Check sheet for the modelled part. Datum: model origin and axes. Units: mm. A direction names the side the tool comes from. Give positions to 0.01 mm unless a question says otherwise; leave off trailing zeros. Write each loop counter-clockwise with the first axis right and the second up, starting at its lowest first coordinate (ties: lowest second). Pieces come first, ordered by that corner, then holes. Notation, with made-up numbers: M 64,85.5 L 111,85.5 A35 cw 111,117.5 Z; hole C 85.25,14 d8. An arc over 180 degrees is marked long. Use CSV: the item, a comma, the result in double quotes. Start each with the question number.
1. Cross-section at A-A, the plane y = 0. Enter the section's corners in (x, z).
2. Cross-section at C-C, the plane z = 34.3. State how many separate pieces and enclosed holes the cut face has, and give its area (3 significant figures).
3. Mould release check, pull along X, two halves, no side actions. Record for faces 3 (the face through (47.7, -40.23, 34.39)), 4 (the face through (44, 0.07, 34.61)), 5 (the face through (-47.7, 40.23, 34.39)), 6 (the face through (44.39, -36.99, 34.61)): +X half, -X half, draft (parallel to the pull), parting line (faces both ways), or undercut.
4. Depth check by flat-ended pin: P1, Ø1.8, axis at x = -45.5, y = 38, coming from the -Z side; P2, Ø0.9, axis at y = 34, z = 35.5, coming from the +X side. Enter the tip coordinate at first touch or a pass-through.
5. Access from +Z, -Z, +X, -X, +Y, -Y to the whole of each face (thin tool, end or side, straight path). Record for faces 1 (the face through (-4, -36, 34.8)), 2 (the face through (-47, 0.07, 34.61)).
6. Scan lines: line 1 (Y direction, x = 45.5, z = 35.35); line 2 (Y direction, x = -45.5, z = 34.85); line 3 (Y direction, x = -37.5, z = 35.45). Record each from-to range of solid material in increasing order.
7. Cross-section at B-B, the plane y = 29. Enter the section's corners in (x, z).
8. Cross-section at D-D, the plane x = -10. Enter the section's corners in (y, z), and give its area (3 significant figures).
from build123d import *

# Parameters (mm, degrees)
PAD011_DEPTH         = 0.8
SKETCH019_W          = 92
SKETCH019_H          = 77
SKETCH019_W_2        = 90
SKETCH019_H_2        = 75
PAD012_DEPTH         = 1.6
SKETCH018_R          = 1.5
POCKET007_DEPTH      = 1.6
POCKET007_DEPTH_BACK = 0.8


with BuildPart() as part:
    # Sketch017 (on XY_Plane002 of Origin004) → Pad011 (new body)
    with BuildSketch(Plane.XY):
        with BuildLine():
            Line((48.3, -38.8), (48.3, 38.8))
            ThreePointArc((48.3, 38.8), (47.714214, 40.214214), (46.3, 40.8))
            Line((46.3, 40.8), (-46.3, 40.8))
            ThreePointArc((-46.3, 40.8), (-47.714214, 40.214214), (-48.3, 38.8))
            Line((-48.3, 38.8), (-48.3, -38.8))
            ThreePointArc((-48.3, -38.8), (-47.714214, -40.214214), (-46.3, -40.8))
            Line((-46.3, -40.8), (46.3, -40.8))
            ThreePointArc((46.3, -40.8), (47.714214, -40.214214), (48.3, -38.8))
        make_face()
        Polygon((-42.5, 35), (42.5, 35), (42.5, -17), (37.5, -17), (37.5, -35), (-37.5, -35), (-37.5, -17), (-42.5, -17), align=None, mode=Mode.SUBTRACT)
    extrude(amount=PAD011_DEPTH)

    # Sketch019 (on XY_Plane002 of Origin004) → Pad012 (join)
    with BuildSketch(Plane.XY):
        Rectangle(SKETCH019_W, SKETCH019_H)
        Rectangle(SKETCH019_W_2, SKETCH019_H_2, mode=Mode.SUBTRACT)
    extrude(amount=PAD012_DEPTH)

    # Sketch018 (on XY_Plane002 of Origin004) → Pocket007 (cut, two sides)
    with BuildSketch(Plane.XY) as pocket007_sk:
        with Locations((-45.5, 38)):
            Circle(SKETCH018_R)
        with Locations((-15.166667, 38)):
            Circle(SKETCH018_R)
        with Locations((15.166667, 38)):
            Circle(SKETCH018_R)
        with Locations((45.5, 29)):
            Circle(SKETCH018_R)
        with Locations((45.5, 0)):
            Circle(SKETCH018_R)
        with Locations((45.5, -38)):
            Circle(SKETCH018_R)
        with Locations((15.166667, -38)):
            Circle(SKETCH018_R)
        with Locations((-15.166667, -38)):
            Circle(SKETCH018_R)
        with Locations((-45.5, -38)):
            Circle(SKETCH018_R)
        with Locations((-45.5, 0)):
            Circle(SKETCH018_R)
    extrude(amount=POCKET007_DEPTH, mode=Mode.SUBTRACT)
    extrude(pocket007_sk.sketch, amount=-POCKET007_DEPTH_BACK, mode=Mode.SUBTRACT)


with BuildPart() as part_1:
    # Body002 placement: moved
    add(part.part.moved(Location((0, 0, 34))))


solid = part_1.part
Worked answers:
1,outline,"M -48.3,34 L -47,34 L -47,34.8 L -48.3,34.8 Z; M -44,34 L -42.5,34 L -42.5,34.8 L -44,34.8 Z; M 42.5,34 L 44,34 L 44,34.8 L 42.5,34.8 Z; M 47,34 L 48.3,34 L 48.3,34.8 L 47,34.8 Z"
2,separate pieces,"1"
2,enclosed holes,"11"
2,area,"2,040 mm^2"
3,face 3,"+X half"
3,face 4,"undercut"
3,face 5,"-X half"
3,face 6,"undercut"
4,P1,"passes through"
4,P2,"stops at x = 46"
5,face 1,"+Z"
5,face 2,"+Z, -Z"
6,line 1,"y = -36.5 to -1.5, 1.5 to 27.5, 30.5 to 38.5"
6,line 2,"y = -36.5 to -1.5, 1.5 to 36.5"
6,line 3,"y = -38.5 to -37.5, 37.5 to 38.5"
7,outline,"M -48.3,34 L -42.5,34 L -42.5,34.8 L -45,34.8 L -45,35.6 L -46,35.6 L -46,34.8 L -48.3,34.8 Z; M 42.5,34 L 44,34 L 44,34.8 L 42.5,34.8 Z; M 47,34 L 48.3,34 L 48.3,34.8 L 47,34.8 Z"
8,outline,"M -40.8,34 L -35,34 L -35,34.8 L -37.5,34.8 L -37.5,35.6 L -38.5,35.6 L -38.5,34.8 L -40.8,34.8 Z; M 35,34 L 40.8,34 L 40.8,34.8 L 38.5,34.8 L 38.5,35.6 L 37.5,35.6 L 37.5,34.8 L 35,34.8 Z"
8,area,"10.9 mm^2"
